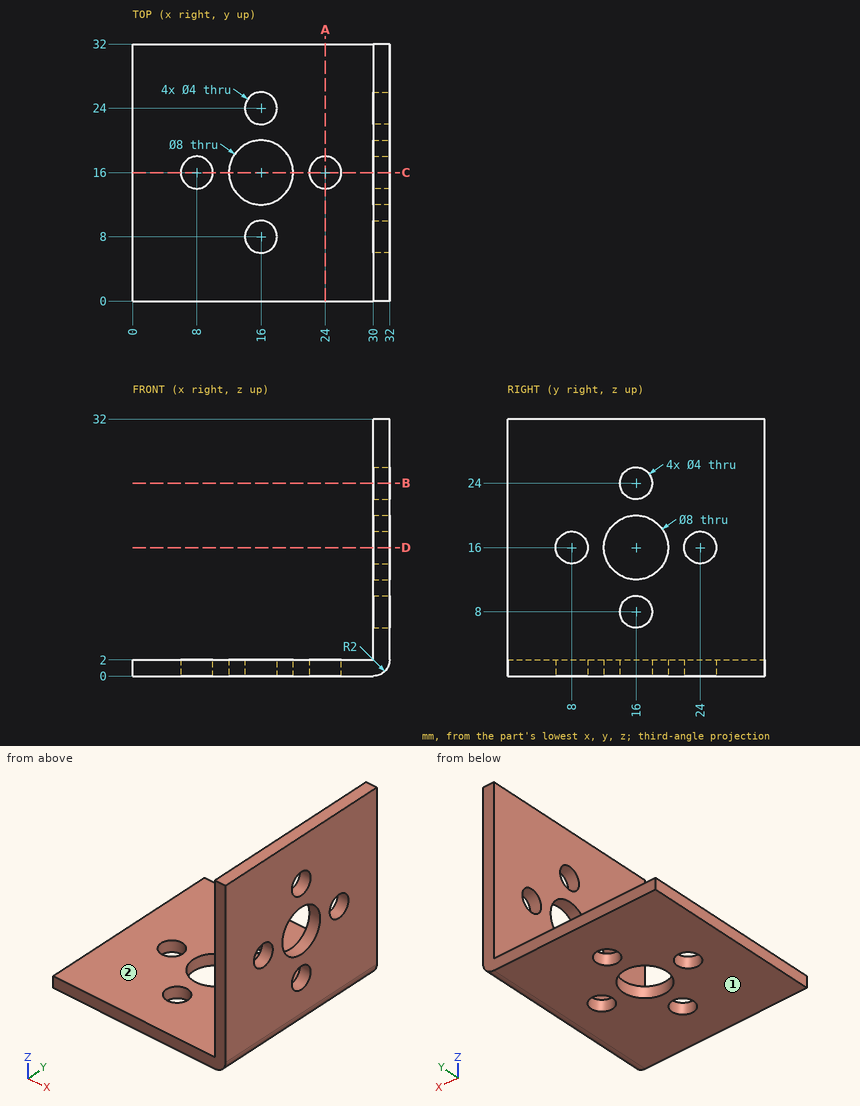
Can you work these out from the drawing? Everything is in mm from the part's minimum corner. A direction names the side the tool comes from. Give positions to 0.01 mm unless a question says otherwise; leave off trailing zeros. Order: outer loops, then holes, each group sorted by start corner. A loop starts at its lowest first (then second) coordinate and runs counter-clockwise, first axis right, second up.
Item 1: If we section it at D-D, the plane z = 16: Write out the boundary of the cut face in (x, y).
Item 2: If we section it at C-C, the plane y = 16: Count the separate pieces of the cut face and the enclosed holes in it, plus the area to 3 significant figures.
Item 3: I need wall thicknesses on line 1 (Y direction, x = 16, z = 1.35); line 2 (Z direction, x = 29, y = 12); line 3 (X direction, y = 5.5, z = 13). Which ranges of each line are inside material? Lowest first, please.
Item 4: For the marked faces 1 and 2, which set-ups out of +Z, -Z, +X, -X, +Y, -Y let a thin tool reach every point of the face, with its end or its side?
Item 5: If we section it at B-B, the plane z = 24: Write out the boundary of the cut face in (x, y), plus the area to 3 significant figures.
Item 6: I'm going to push flat-ended pins straight in: pin 1 (6.5 mm diameter, centred on x = 24, y = 16, fed in from -Z); pin 2 (9 mm diameter, centred on y = 23.5, z = 24, fed in from -X); pin 3 (15 mm diameter, centred on x = 16.5, y = 22.5, fed in from +Z). Where does each tip first touch, or does it pass through?
Item 7: If we section it at A-A, the plane x = 24: Write out the boundary of the cut face in (y, z).
Values:
1. outline: (30, 0) - (32, 0) - (32, 6) - (30, 6) - close; (30, 10) - (32, 10) - (32, 12) - (30, 12) - close; (30, 20) - (32, 20) - (32, 22) - (30, 22) - close; (30, 26) - (32, 26) - (32, 32) - (30, 32) - close
2. separate pieces: 7
2. enclosed holes: 0
2. area: 59.1 mm2
3. line 1: y = 0 to 6, 10 to 12, 20 to 22, 26 to 32
3. line 2: z = 0 to 2
3. line 3: x = 30 to 32
4. face 1: -Z, +X, -X, +Y, -Y
4. face 2: +Z, -X, +Y, -Y
5. outline: (30, 0) - (32, 0) - (32, 14) - (30, 14) - close; (30, 18) - (32, 18) - (32, 32) - (30, 32) - close
5. area: 56.0 mm2
6. pin 1: stops at z = 0
6. pin 2: stops at x = 30
6. pin 3: stops at z = 2
7. outline: (0, 0) - (14, 0) - (14, 2) - (0, 2) - close; (18, 0) - (32, 0) - (32, 2) - (18, 2) - close
